Check sheet for the modelled part. Datum: model origin and axes. Units: mm. A direction names the side the tool comes from. Round coordinates to 2 decimals unless told otherwise and drop trailing zeros. Write each loop counter-clockwise with the first axis right and the second up, starting at its lowest first coordinate (ties: lowest second). Pieces come first, ordered by that corner, then holes. Notation, with made-up numbers: (82.25, -16) -> (138.25, -16) arc R26 cw to (138.25, 15) -> close; hole circle Ø8 at (58.25, 23). An arc over 180 degrees is marked (long way). One line per item, written item: value.
from build123d import *

# Parameters (mm, degrees)
SKETCH1_W           = 304.8
SKETCH1_H           = 304.8
BOSS_EXTRUDE1_DEPTH = 2.54
SKETCH2_W           = 304.8
SKETCH2_H           = 304.8
SKETCH2_W_2         = 299.72
SKETCH2_H_2         = 299.72
BOSS_EXTRUDE2_DEPTH = 19.05
FILLET1_R           = 2.54


with BuildPart() as part:
    # Sketch1 → Boss-Extrude1 (new body)
    with BuildSketch(Plane.XY):
        Rectangle(SKETCH1_W, SKETCH1_H)
    extrude(amount=BOSS_EXTRUDE1_DEPTH)

    # Sketch2 → Boss-Extrude2 (add)
    with BuildSketch(Plane.XY.offset(2.54)):
        Rectangle(SKETCH2_W, SKETCH2_H)
        Rectangle(SKETCH2_W_2, SKETCH2_H_2, mode=Mode.SUBTRACT)
    extrude(amount=-BOSS_EXTRUDE2_DEPTH)

    # Fillet1
    fillet1_edges = [part.edges().sort_by_distance(p)[0] for p in [
        (-152.4, 0, 2.54),
        (0, -152.4, 2.54),
        (0, -149.86, -16.51),
        (152.4, 0, 2.54),
        (0, 152.4, 2.54),
    ]]
    fillet(fillet1_edges, radius=FILLET1_R - 0.0001)  # a hair under: the kernel refuses the full size


solid = part.part
Item 1: Release check for a two-part mould opening along Y. For faces 3 (the flat face through (152.4, -2, -8)), 4 (the flat face through (-2, 149.86, -8)), 5 (the flat face through (-2, 152.4, -8)), 6 (the flat face through (-2, -149.86, -7)) record: pulls with the +Y half, pulls with the -Y half, needs draft (parallel to the pull), parting line crosses it, or undercut.
Result set:
face 3: needs draft
face 4: undercut
face 5: pulls with the +Y half
face 6: undercut
Item 2: Material ranges on line 1 along Y through (x, z) = (19, -9); line 2 along Z through (x, y) = (-13, -87), recorded low to high.
Result set:
line 1: -152.4 to -149.86, 149.86 to 152.4
line 2: 0 to 2.54
Item 3: Sectioned sample at B-B (y = 22). Enter the section's corners in (x, z), then the cut area to 3 significant figures.
Result set:
outline: (-152.4, -16.51) -> (-149.86, -16.51) -> (-149.86, 0) -> (149.86, 0) -> (149.86, -16.51) -> (152.4, -16.51) -> (152.4, 0) arc R2.54 ccw to (149.86, 2.54) -> (-149.86, 2.54) arc R2.54 ccw to (-152.4, 0) -> close
area: 855 mm^2
Item 4: Sectioned sample at A-A (z = -10.25). Enter the section's corners in (x, y), then the cut area to 3 significant figures.
Result set:
outline: (-152.4, -152.4) -> (152.4, -152.4) -> (152.4, 152.4) -> (-152.4, 152.4) -> close; hole (-149.86, -149.86) -> (149.86, -149.86) -> (149.86, 149.86) -> (-149.86, 149.86) -> close
area: 3,070 mm^2
Item 5: Depth check by flat-ended pin: pin 1 (5 mm diameter, centred on x = 15.5, y = -107, fed in from -Z). Enter the tip coordinate at first touch or a pass-through.
Result set:
pin 1: z = 0
Item 6: Tool access check on faces 1 (the flat face through (-2, 2, 2.54)), 2 (the flat face through (149.86, -3, -8)). Record the directions out of +Z, -Z, +X, -X, +Y, -Y that give a thin tool (end or side, any length) a straight path to the whole face; none if there is none.
Result set:
face 1: +Z, +X, -X, +Y, -Y
face 2: -Z
